```python
from build123d import *

# Parameters (mm, degrees)
SKETCH1_W           = 21.95
SKETCH1_H           = 16
BOSS_EXTRUDE1_DEPTH = 2
SKETCH2_W           = 3
SKETCH2_H           = 16
BOSS_EXTRUDE2_DEPTH = 12.4
SKETCH3_W           = 3
SKETCH3_H           = 16
BOSS_EXTRUDE3_DEPTH = 8
SKETCH4_W           = 3
SKETCH4_H           = 16
BOSS_EXTRUDE4_DEPTH = 8
SKETCH5_R           = 1
CUT_EXTRUDE1_DEPTH  = 8
FILLET1_R           = 2
FILLET2_R           = 2


with BuildPart() as part:
    # Sketch1 → Boss-Extrude1 (new body)
    with BuildSketch(Plane.XY):
        with Locations((10.975, 8)):
            Rectangle(SKETCH1_W, SKETCH1_H)
    extrude(amount=BOSS_EXTRUDE1_DEPTH)

    # Sketch2 → Boss-Extrude2 (add)
    with BuildSketch(Plane.XY.offset(2)):
        with Locations((1.5, 8)):
            Rectangle(SKETCH2_W, SKETCH2_H)
        with Locations((20.45, 8)):
            Rectangle(SKETCH2_W, SKETCH2_H)
    extrude(amount=BOSS_EXTRUDE2_DEPTH)

    # Sketch3 → Boss-Extrude3 (add)
    with BuildSketch(Plane(origin=(21.95, 0, 0), x_dir=(0, 0, -1), z_dir=(1, 0, 0))):
        with Locations((-12.9, 8)):
            Rectangle(SKETCH3_W, SKETCH3_H)
    extrude(amount=BOSS_EXTRUDE3_DEPTH)

    # Sketch4 → Boss-Extrude4 (add)
    with BuildSketch(Plane.ZY):
        with Locations((12.9, 8)):
            Rectangle(SKETCH4_W, SKETCH4_H)
    extrude(amount=BOSS_EXTRUDE4_DEPTH)

    # Sketch5 → Cut-Extrude1 (cut)
    with BuildSketch(Plane(origin=(0, 0, 11.4), x_dir=(-1, 0, 0), z_dir=(0, 0, -1))):
        with Locations((4, 4)):
            Circle(SKETCH5_R)
        with Locations((-25.95, 4)):
            Circle(SKETCH5_R)
        with Locations((4, 12)):
            Circle(SKETCH5_R)
        with Locations((-25.95, 12)):
            Circle(SKETCH5_R)
    extrude(amount=-CUT_EXTRUDE1_DEPTH, mode=Mode.SUBTRACT)

    # Fillet1
    fillet1_edges = [part.edges().sort_by_distance(p)[0] for p in [
        (3, 8, 2),
        (18.95, 8, 2),
    ]]
    fillet(fillet1_edges, radius=FILLET1_R)

    # Fillet2
    fillet2_edges = [part.edges().sort_by_distance(p)[0] for p in [
        (21.95, 8, 0),
        (0, 8, 0),
    ]]
    fillet(fillet2_edges, radius=FILLET2_R)


solid = part.part
```
The listing builds one solid part. Answer for the finished solid, in the listing's coordinates (mm). A direction names the side the tool comes from. Coordinates: 2 decimals unless noted, no trailing zeros. Loops run counter-clockwise (first coordinate to the right, second up) from the corner with the lowest first, then second, coordinate; pieces in that order, holes last. Notation, with made-up numbers: (74.25, 2.5) - (83.25, 2.5) arc R11 cw to (83.25, 23.5) - close; hole circle Ø3 at (-33.5, 43). An arc over 180 degrees is marked (long way). Use a Markdown table: item, result. Add a question column.
1) For faces 4 (the flat face through (11, 8, 2)), 5 (the flat face through (0, 8, 7)), 6 (the flat face through (21.95, 8, 7)), determine the directions among +Z, -Z, +X, -X, +Y, -Y from which every point of the face is accessible in a straight line to the end or side of a thin tool.
2) The part is cut by section B-B, the plane z = 13.25. Give the vertices of the cut face in (x, y).
3) Find the intervals of material crossed by line 1 (Y direction, x = -4, z = 13.25); line 2 (X direction, y = 5.5, z = 4.25); line 3 (X direction, y = 1.5, z = 13.75), in increasing order.
4) The part is cut by section C-C, the plane x = 25.95. Give the vertices of the cut face in (y, z), and give its area (3 significant figures).
5) The mould has two halves that part along Y. Classify faces 1 (the cylindrical face through (26.95, 12.04, 12.88)), 2 (the flat face through (11, 8, 0)), 3 (the flat face through (12.5, 0, 1.8)): released by +Y, released by -Y, zero draft, split by the parting line, or undercut.
6) The part is cut by section A-A, the plane y = 4. Give the vertices of the cut face in (x, z), and give its area (3 significant figures).
7) Given pin 1 (6.5 mm diameter, centred on x = 25.5, y = 11.5, fed in from -Z); pin 2 (1.2 mm diameter, centred on x = 25.95, y = 12, fed in from +Z); pin 3 (4 mm diameter, centred on x = -1, y = 5, fed in from -Z); pin 4 (6 mm diameter, centred on y = 6.5, z = 8, fed in from +X), each flat-ended and moving along its own axis, determine where each tip first touches the part or whether it passes through.
8) The part is cut by section D-D, the plane z = 7.5. Give the vertices of the cut face in (x, y), and give its area (3 significant figures).
Here are the results:
| question | item | result |
|---|---|---|
| 1 | face 4 | +Z, +Y, -Y |
| 1 | face 5 | -Z, -X, +Y, -Y |
| 1 | face 6 | -Z, +X, +Y, -Y |
| 2 | outline | (-8, 0) - (3, 0) - (3, 16) - (-8, 16) - close; (18.95, 0) - (29.95, 0) - (29.95, 16) - (18.95, 16) - close; hole circle Ø2 at (-4, 4); hole circle Ø2 at (-4, 12); hole circle Ø2 at (25.95, 4); hole circle Ø2 at (25.95, 12) |
| 3 | line 1 | y = 0 to 3, 5 to 11, 13 to 16 |
| 3 | line 2 | x = 0 to 3, 18.95 to 21.95 |
| 3 | line 3 | x = -8 to 3, 18.95 to 29.95 |
| 4 | outline | (0, 11.4) - (3, 11.4) - (3, 14.4) - (0, 14.4) - close; (5, 11.4) - (11, 11.4) - (11, 14.4) - (5, 14.4) - close; (13, 11.4) - (16, 11.4) - (16, 14.4) - (13, 14.4) - close |
| 4 | area | 36.0 mm^2 |
| 5 | face 1 | undercut |
| 5 | face 2 | zero draft |
| 5 | face 3 | released by -Y |
| 6 | outline | (-8, 11.4) - (-5, 11.4) - (-5, 14.4) - (-8, 14.4) - close; (-3, 11.4) - (0, 11.4) - (0, 2) arc R2 ccw to (2, 0) - (19.95, 0) arc R2 ccw to (21.95, 2) - (21.95, 11.4) - (24.95, 11.4) - (24.95, 14.4) - (18.95, 14.4) - (18.95, 4) arc R2 cw to (16.95, 2) - (5, 2) arc R2 cw to (3, 4) - (3, 14.4) - (-3, 14.4) - close; (26.95, 11.4) - (29.95, 11.4) - (29.95, 14.4) - (26.95, 14.4) - close |
| 6 | area | 154 mm^2 |
| 7 | pin 1 | stops at z = 11.4 |
| 7 | pin 2 | passes through |
| 7 | pin 3 | stops at z = 0.27 |
| 7 | pin 4 | stops at x = 21.95 |
| 8 | outline | (0, 0) - (3, 0) - (3, 16) - (0, 16) - close; (18.95, 0) - (21.95, 0) - (21.95, 16) - (18.95, 16) - close |
| 8 | area | 96.0 mm^2 |
